Verification items for this drawing (mm, ordinates from the low corner). A direction names the side the tool comes from. Coordinates: 2 decimals unless noted, no trailing zeros. Loops run counter-clockwise (first coordinate to the right, second up) from the corner with the lowest first, then second, coordinate; pieces in that order, holes last. Notation, with made-up numbers: (20.5, 70.25) - (25.5, 70.25) arc R11 ccw to (25.5, 87.25) - close; hole circle Ø2 at (18.25, -9.5). An arc over 180 degrees is marked (long way). Write each question's results on one line, items separated by ' | '. Start each with the question number.
(1) Go/stop test with flat-tipped pins: pin 1 Ø4 at (x, y) = (5.5, 13) entering from +Z; pin 2 Ø5 at (x, z) = (17, 5.5) entering from -Y; pin 3 Ø13 at (x, y) = (37.5, 10.5) entering from -Z. Record where each tip stops, or that it passes through.
(2) Sectioned sample at B-B (y = 24.25). Enter the section's corners in (x, z).
(3) Material ranges on probe 1 along X at (y, z) = (13, 12.25); probe 2 along X at (y, z) = (24.5, 8); probe 3 along X at (y, z) = (22.05, 6.5), recorded low to high.
(4) Mould release check, pull along X, two halves, no side actions. Record for the marked faces 1, 2 and 3: pulls with the +X half, pulls with the -X half, needs draft (parallel to the pull), parting line crosses it, or undercut.
(5) Sectioned sample at D-D (x = 17.5). Enter the section's corners in (y, z).
(6) Sectioned sample at A-A (y = 13). Enter the section's corners in (x, z).
(7) Sectioned sample at C-C (z = 7.5). Enter the section's corners in (x, y).
(8) Access from +Z, -Z, +X, -X, +Y, -Y to the whole of each face (thin tool, end or side, straight path). Record for the marked faces 4, 5 and 6.
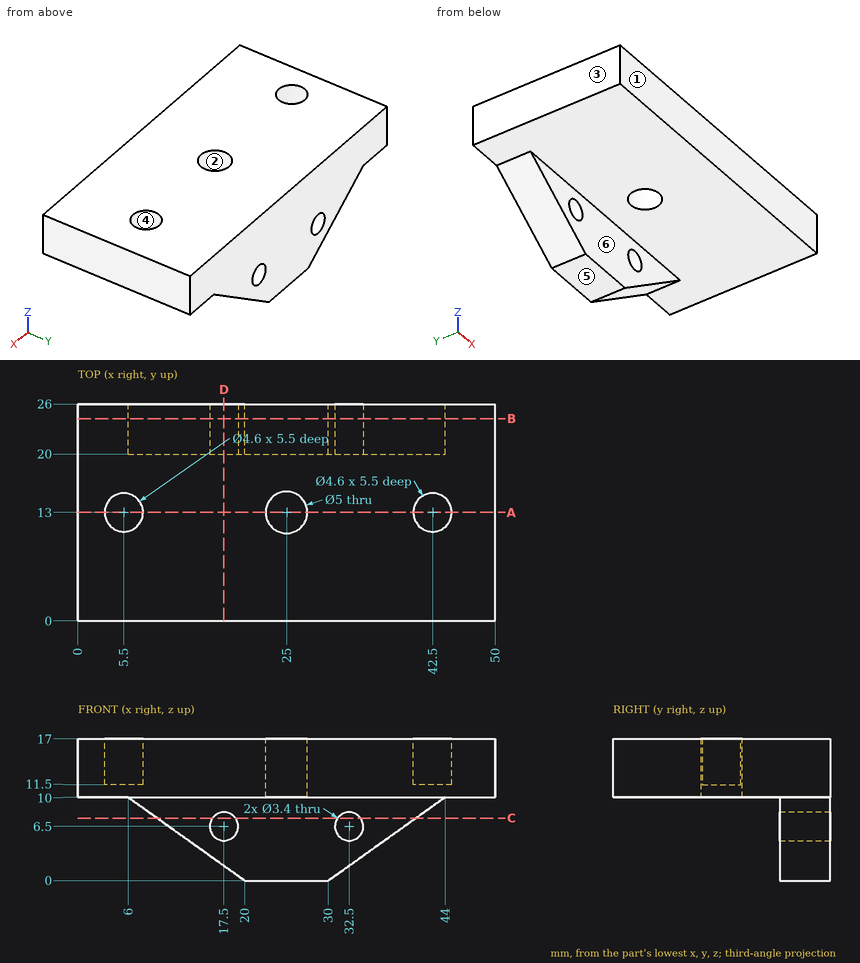
Outcome:
1) pin 1: stops at z = 11.5 | pin 2: stops at y = 20 | pin 3: stops at z = 10
2) outline: (0, 10) - (6, 10) - (20, 0) - (30, 0) - (44, 10) - (50, 10) - (50, 17) - (0, 17) - close; hole circle Ø3.4 at (17.5, 6.5); hole circle Ø3.4 at (32.5, 6.5)
3) probe 1: x = 0 to 3.2, 7.8 to 22.5, 27.5 to 40.2, 44.8 to 50 | probe 2: x = 8.8 to 16.7, 18.3 to 31.7, 33.3 to 41.2 | probe 3: x = 10.9 to 15.8, 19.2 to 30.8, 34.2 to 39.1
4) face 1: needs draft | face 2: undercut | face 3: pulls with the -X half
5) outline: (0, 10) - (20, 10) - (20, 8.2) - (26, 8.2) - (26, 17) - (0, 17) - close; (20, 1.79) - (26, 1.79) - (26, 4.8) - (20, 4.8) - close
6) outline: (0, 10) - (22.5, 10) - (22.5, 17) - (7.8, 17) - (7.8, 11.5) - (3.2, 11.5) - (3.2, 17) - (0, 17) - close; (27.5, 10) - (50, 10) - (50, 17) - (44.8, 17) - (44.8, 11.5) - (40.2, 11.5) - (40.2, 17) - (27.5, 17) - close
7) outline: (9.5, 20) - (16.13, 20) - (16.13, 26) - (9.5, 26) - close; (18.87, 20) - (31.13, 20) - (31.13, 26) - (18.87, 26) - close; (33.87, 20) - (40.5, 20) - (40.5, 26) - (33.87, 26) - close
8) face 4: +Z | face 5: -Z, +X, -X, +Y, -Y | face 6: -Z, +X, -X, -Y
